Design review of the part built by this model. Coordinates are the model's own, in mm. A direction names the side the tool comes from. Give positions to 0.01 mm unless a question says otherwise; leave off trailing zeros. Loops run counter-clockwise (first coordinate to the right, second up) from the corner with the lowest first, then second, coordinate; pieces in that order, holes last. Notation, with made-up numbers: M 34,57.5 L 51,57.5 A25 cw 51,88.5 Z; hole C 71.5,-21 d3. An arc over 180 degrees is marked long. Answer as CSV lines item,"result".
```python
from build123d import *

# Parameters (mm, degrees)
SKETCH1_R                 = 16
SKETCH1_R_2               = 13
BOTTOM_RING_BAYONET_DEPTH = 8
SKETCH2_R                 = 16
SKETCH2_R_2               = 14.4
WELL_TUBE_DEPTH           = 65.7
SKETCH3_R                 = 19
SKETCH3_R_2               = 14.9
HATCH_FLANGE_DEPTH        = 1.2
SKETCH4_R                 = 1.6
BAYONET_PIN_STBD_DEPTH    = 3.6
SKETCH5_R                 = 1.6
BAYONET_PIN_PORT_DEPTH    = 3.6


with BuildPart() as part:
    # Sketch1 → Bottom_ring_bayonet (new body)
    with BuildSketch(Plane.XY.offset(-12)):
        with Locations((48, 0)):
            Circle(SKETCH1_R)
        with Locations((48, 0)):
            Circle(SKETCH1_R_2, mode=Mode.SUBTRACT)
    extrude(amount=BOTTOM_RING_BAYONET_DEPTH)

    # Sketch2 → Well_tube (add)
    with BuildSketch(Plane.XY.offset(-4)):
        with Locations((48, 0)):
            Circle(SKETCH2_R)
        with Locations((48, 0)):
            Circle(SKETCH2_R_2, mode=Mode.SUBTRACT)
    extrude(amount=WELL_TUBE_DEPTH)

    # Sketch3 → Hatch_flange (add)
    with BuildSketch(Plane.XY.offset(60.6)):
        with Locations((48, 0)):
            Circle(SKETCH3_R)
        with Locations((48, 0)):
            Circle(SKETCH3_R_2, mode=Mode.SUBTRACT)
    extrude(amount=HATCH_FLANGE_DEPTH)

    # Sketch4 → Bayonet_pin_stbd (add)
    with BuildSketch(Plane(origin=(0, 15, 0), x_dir=(1, 0, 0), z_dir=(0, 1, 0))):
        with Locations(Location((48, 7, 0), (0, 0, 90))):
            Circle(SKETCH4_R)
    extrude(amount=BAYONET_PIN_STBD_DEPTH)

    # Sketch5 → Bayonet_pin_port (add)
    with BuildSketch(Plane(origin=(0, -18.6, 0), x_dir=(1, 0, 0), z_dir=(0, 1, 0))):
        with Locations(Location((48, 7, 0), (0, 0, 90))):
            Circle(SKETCH5_R)
    extrude(amount=BAYONET_PIN_PORT_DEPTH)


solid = part.part
```
1. We need section B-B, the plane y = 0. Write out the cut boundary in (x, z), plus the area to 3 significant figures.
Answer block:
outline,"M 29,60.6 L 32,60.6 L 32,-12 L 35,-12 L 35,-4 L 33.6,-4 L 33.6,61.7 L 33.1,61.7 L 33.1,61.8 L 29,61.8 Z; M 61,-12 L 64,-12 L 64,60.6 L 67,60.6 L 67,61.8 L 62.9,61.8 L 62.9,61.7 L 62.4,61.7 L 62.4,-4 L 61,-4 Z"
area,"266 mm²"
2. The part is to be moulded in two halves that separate along X. For faces 5 (the cylindrical face through (35.013, 0.572, -8.056)), 6 (the cylindrical face through (49.42, -17.28, -7.74)), 7 (the cylindrical face through (61.735, 4.325, 28.39)), 8 (the flat face through (48, -18.6, -7)), say which applies: pulls with the +X half, pulls with the -X half, needs draft (parallel to the pull), parting line crosses it, or undercut.
Answer block:
face 5,"undercut"
face 6,"parting line crosses it"
face 7,"undercut"
face 8,"needs draft"
3. To check wall thickness, follow L1, parallel to Y at x = 48, z = -9; L2, parallel to Y at x = 47.5, z = 53.5; L3, parallel to X at y = 5.5, z = 58. State the ranges of each line that lie inside material, in increasing order. Write a range as [from, to].
Answer block:
L1,"[-16, -13], [13, 16]"
L2,"[-15.99, -14.39], [14.39, 15.99]"
L3,"[32.98, 34.69], [61.31, 63.02]"
4. We need section C-C, the plane z = -7. Write out the cut boundary in (x, y), plus the area to 3 significant figures.
Answer block:
outline,"M 46.4,-18.6 L 49.6,-18.6 L 49.6,-15.92 A16 ccw 49.6,15.92 L 49.6,18.6 L 46.4,18.6 L 46.4,15.92 A16 ccw 46.4,-15.92 Z; hole C 48,0 d26"
area,"290 mm²"
5. For faces 1 (the flat face through (48, 18.6, -7)), 2 (the cylindrical face through (43.881, -18.548, 61.192)), 3 (the flat face through (46, 13, -4)), 4 (the cylindrical face through (49.42, 17.24, -7.74)), list the 3-axis set-ups (+Z, -Z, +X, -X, +Y, -Y) from which the entire face can be reached by the end or side of a thin tool; tool diameter is ignored.
Answer block:
face 1,"-Z, +X, -X, +Y"
face 2,"+Z, -Z"
face 3,"+Z"
face 4,"+Y"
6. We need section D-D, the plane y = 8.5. Write out the cut boundary in (x, z), plus the area to 3 significant figures.
Answer block:
outline,"M 31.01,60.6 L 34.44,60.6 L 34.44,-12 L 38.16,-12 L 38.16,-4 L 36.38,-4 L 36.38,61.7 L 35.76,61.7 L 35.76,61.8 L 31.01,61.8 Z; M 57.84,-12 L 61.56,-12 L 61.56,60.6 L 64.99,60.6 L 64.99,61.8 L 60.24,61.8 L 60.24,61.7 L 59.62,61.7 L 59.62,-4 L 57.84,-4 Z"
area,"322 mm²"
7. We need section A-A, the plane x = 48. Write out the cut boundary in (y, z).
Answer block:
outline,"M -19,60.6 L -16,60.6 L -16,-5.4 L -18.6,-5.4 L -18.6,-8.6 L -16,-8.6 L -16,-12 L -13,-12 L -13,-4 L -14.4,-4 L -14.4,61.7 L -14.9,61.7 L -14.9,61.8 L -19,61.8 Z; M 13,-12 L 16,-12 L 16,-8.6 L 18.6,-8.6 L 18.6,-5.4 L 16,-5.4 L 16,60.6 L 19,60.6 L 19,61.8 L 14.9,61.8 L 14.9,61.7 L 14.4,61.7 L 14.4,-4 L 13,-4 Z"
8. For P1, Ø12, axis at x = 54.5, z = -4.5, coming from the -Y side; P2, Ø21, axis at x = 48, y = 0, coming from the -Z side; P3, Ø2.5, axis at x = 48.5, z = -7, coming from the +Y side; P4, Ø3, axis at x = 33, z = 29.5, coming from the -Y side, all flat-tipped, find the tip position at first contact; note any pin that passes through.
Answer block:
P1,"y = -18.6"
P2,"through"
P3,"y = 18.6"
P4,"y = -8.59"
